Design review of the part built by this model. Coordinates are the model's own, in mm. Face numbers are marked on the shaded views. A direction names the side the tool comes from. Give positions to 0.01 mm unless a question says otherwise; leave off trailing zeros. Loops run counter-clockwise (first coordinate to the right, second up) from the corner with the lowest first, then second, coordinate; pieces in that order, holes last. Notation, with made-up numbers: (-7.5, -36) -> (27.5, -36) arc R33 ccw to (27.5, 3) -> close; hole circle Ø8 at (12, 14.5). An arc over 180 degrees is marked (long way). Use CSV: the item, a comma, the result in double quotes. Start each with the question number.
Item 1: We need section A-A (y = 3.75). Count the separate pieces of the cut face and the enclosed holes in it, plus the area to 3 significant figures.
Item 2: For the marked faces 1 and 2, list the 3-axis set-ups (+Z, -Z, +X, -X, +Y, -Y) from which the entire face can be reached by the end or side of a thin tool; tool diameter is ignored.
Item 3: Wall thickness on line 1 along Z through (x, y) = (3, 2.25); line 2 along X through (y, z) = (5, 3); line 3 along Y through (x, z) = (-9.5, 6.5): over which ranges is each line inside the solid? List them lowest first. Write a range as from..to.
Item 4: Clearance check with flat-ended pins moving along their axes: pin 1 (4 mm diameter, centred on x = -9, z = 0.5, fed in from -Y); pin 2 (5 mm diameter, centred on x = 4.5, z = -3.5, fed in from +Y); pin 3 (6 mm diameter, centred on x = -4.37, z = -3.18, fed in from +Y); pin 4 (1 mm diameter, centred on x = 5, z = -1, fed in from +Y). State where each tip first meets the part, or that it passes through.
Item 5: The part is to be moulded in two halves that separate along Z. For the marked faces 3, 4, 5 and 6, say which applies: +Z half, -Z half, draft (parallel to the pull), parting line (faces both ways), or undercut.
Item 6: We need section B-B (z = 3.25). State the section outline as (x, y) points, plus the area to 3 significant figures.
from build123d import *

# Parameters (mm, degrees)
SKETCH1_W                                         = 25.4
SKETCH1_H                                         = 15.875
BOSS_EXTRUDE1_DEPTH                               = 6.35
CHAMFER1_SIZE                                     = 6.35
CUT_EXTRUDE1_DEPTH                                = 6.746875
SKETCH3_R                                         = 1.63195
CUT_EXTRUDE2_DEPTH                                = 17.267034341
CSK_FOR_8_FLAT_HEAD_MACHINE_SCREW_100_D           = 4.4958
CSK_FOR_8_FLAT_HEAD_MACHINE_SCREW_100_CSINK_D     = 8.4328
CSK_FOR_8_FLAT_HEAD_MACHINE_SCREW_100_CSINK_ANGLE = 100


with BuildPart() as part:
    # Sketch1 → Boss-Extrude1 (new body)
    with BuildSketch(Plane(origin=(0, 0, 0), x_dir=(1, 0, 0), z_dir=(0, 1, 0))):
        Rectangle(SKETCH1_W, SKETCH1_H)
    extrude(amount=BOSS_EXTRUDE1_DEPTH)

    # Chamfer1
    chamfer1_edges = [part.edges().sort_by_distance(p)[0] for p in [
        (-12.7, 3.175, -7.9375),
        (12.7, 3.175, -7.9375),
    ]]
    chamfer(chamfer1_edges, length=CHAMFER1_SIZE)

    # Sketch2 → Cut-Extrude1 (cut)
    with BuildSketch(Plane.XY.offset(7.9375)):
        with BuildLine():
            Line((-12.7, 2.030696103), (-12.7, 0))
            Line((-12.7, 0), (12.7, 0))
            Line((12.7, 0), (12.7, 2.030696103))
            ThreePointArc((12.7, 2.030696103), (0, 3.096482857), (-12.7, 2.030696103))
        make_face()
    extrude(amount=-CUT_EXTRUDE1_DEPTH, mode=Mode.SUBTRACT)

    # Sketch3 → Cut-Extrude2 (cut, through all)
    with BuildSketch(Plane(origin=(0, 6.35, 0), x_dir=(1, 0, 0), z_dir=(0, 1, 0))):
        with Locations(Location((0, -4.129280278, 0), (0, 0, 270))):
            Circle(SKETCH3_R)
    extrude(amount=-CUT_EXTRUDE2_DEPTH, mode=Mode.SUBTRACT)

    # CSK for #8 Flat Head Machine Screw (100)1 (through all)
    with Locations(Plane(origin=(0, 6.35, 0), x_dir=(1, 0, 0), z_dir=(0, 1, 0))):
        with Locations((-4.365625, 3.175), (4.365625, 3.175)):
            CounterSinkHole(CSK_FOR_8_FLAT_HEAD_MACHINE_SCREW_100_D / 2, CSK_FOR_8_FLAT_HEAD_MACHINE_SCREW_100_CSINK_D / 2, counter_sink_angle=CSK_FOR_8_FLAT_HEAD_MACHINE_SCREW_100_CSINK_ANGLE)


solid = part.part
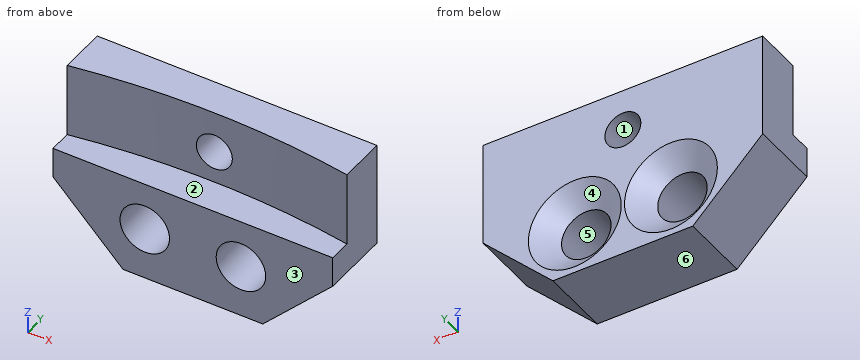
Results found:
1,separate pieces,"1"
1,enclosed holes,"3"
1,area,"323 mm²"
2,face 1,"+Y, -Y"
2,face 2,"+Z, -Y"
3,line 1,"-7.94..-4.96, -1.39..1.19"
3,line 2,"-12.7..-1.18, 1.18..12.7"
3,line 3,"2.5..6.35"
4,pin 1,"y = 0"
4,pin 2,"y = 5.2"
4,pin 3,"y = 5.33"
4,pin 4,"y = 5.13"
5,face 3,"draft"
5,face 4,"undercut"
5,face 5,"undercut"
5,face 6,"-Z half"
6,outline,"(-12.7, 2.03) arc R76.2 cw to (-1.37, 3.08) -> (-1.37, 6.35) -> (-12.7, 6.35) -> close; (1.37, 3.08) arc R76.2 cw to (12.7, 2.03) -> (12.7, 6.35) -> (1.37, 6.35) -> close"
6,area,"82.7 mm²"
